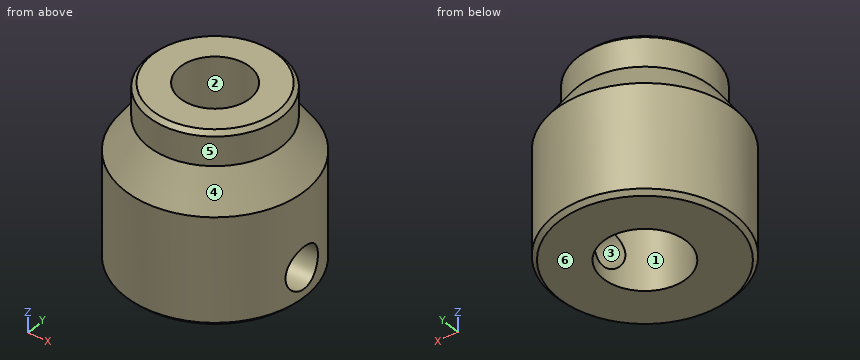
```python
from build123d import *

# Parameters (mm, degrees)
CONNECTOR_M5X0_8_TAPPED_HOLE_D        = 4.2
CONNECTOR_M5X0_8_TAPPED_HOLE_DEPTH    = 7.4
CONNECTOR_M5X0_8_TAPPED_HOLE_TIP      = 1.2618073
SET_SCREW_1_M3X0_5_TAPPED_HOLE_REACH  = 16.767
SET_SCREW_1_M3X0_5_TAPPED_HOLE_BORE_R = 1.25
EDGE_CHAMFERS_SIZE                    = 0.25


with BuildPart() as part:
    # Body Sketch → Body Revolve (revolve)
    with BuildSketch(Plane(origin=(0, 0, 0), x_dir=(-1, 0, 0), z_dir=(0, 1, 0))):
        Polygon((1, 10.5), (4, 10.5), (4, 8.5), (5.4, 6.5), (5.4, 0), (2.5, 0), (2.5, 6), (1, 6), align=None)
    revolve(axis=Axis((0, 0, 0), (0, 0, 1)))

    # Connector M5x0.8 Tapped Hole
    with Locations(Plane.XY.offset(10.5)):
        with Locations((0, 0)):
            Hole(CONNECTOR_M5X0_8_TAPPED_HOLE_D / 2, depth=CONNECTOR_M5X0_8_TAPPED_HOLE_DEPTH)
            with Locations((0, 0, -(CONNECTOR_M5X0_8_TAPPED_HOLE_DEPTH + CONNECTOR_M5X0_8_TAPPED_HOLE_TIP / 2))):  # 118° drill point
                Cone(0, CONNECTOR_M5X0_8_TAPPED_HOLE_D / 2, CONNECTOR_M5X0_8_TAPPED_HOLE_TIP, mode=Mode.SUBTRACT)

    # Set Screw 1 M3x0.5 Tapped Hole bore (on position points) → Set Screw 1 M3x0.5 Tapped Hole (cut, up to next)
    with BuildSketch(Plane(origin=(5.4, 0, 2), x_dir=(0, 1, 0), z_dir=(1, 0, 0)), mode=Mode.PRIVATE) as set_screw_1_m3x0_5_tapped_hole_sk1:
        Circle(SET_SCREW_1_M3X0_5_TAPPED_HOLE_BORE_R)
    set_screw_1_m3x0_5_tapped_hole_tool1 = extrude(set_screw_1_m3x0_5_tapped_hole_sk1.sketch, amount=-SET_SCREW_1_M3X0_5_TAPPED_HOLE_REACH, mode=Mode.PRIVATE) & part.part
    add(set_screw_1_m3x0_5_tapped_hole_tool1.solids().sort_by_distance((5.4, 0, 2))[0], mode=Mode.SUBTRACT)

    # Edge Chamfers
    edge_chamfers_edges = [part.edges().sort_by_distance(p)[0] for p in [
        (5.4, 0, 0),
        (4, 0, 10.5),
    ]]
    chamfer(edge_chamfers_edges, length=EDGE_CHAMFERS_SIZE)


solid = part.part
```
Build history of the part. All positions in model axes, mm. Face numbers are marked on the shaded views. A direction names the side the tool comes from. Give positions to 0.01 mm unless a question says otherwise; leave off trailing zeros. Loops run counter-clockwise (first coordinate to the right, second up) from the corner with the lowest first, then second, coordinate; pieces in that order, holes last.
1) Band-saw the part on D-D on z = 2. List the corners of the cut face in (x, y).
Values follow:
outline: (2.17, -1.25) arc R2.5 cw (long way) to (2.17, 1.25) - (5.25, 1.25) arc R5.4 ccw (long way) to (5.25, -1.25) - close
2) Drop flat-ended pins along their axis: P1, Ø5, axis at x = -2.5, z = 2, coming from the +Y side; P2, Ø3, axis at y = -4, z = 1.5, coming from the +X side; P3, Ø1, axis at x = 3.5, y = -3.5, coming from the +Z side; P4, Ø6, axis at x = -4, z = 9.5, coming from the +Y side. Give the stop position or say it passes through.
Values follow:
P1: stops at y = 5.4
P2: stops at x = 4.79
P3: stops at z = 7.86
P4: stops at y = 4.47
3) Two-plate mould, pull along X, no slides. Class the marked faces 1, 2, 3 and 4: released by +X, released by -X, zero draft, split by the parting line, or undercut.
Values follow:
face 1: undercut
face 2: undercut
face 3: zero draft
face 4: split by the parting line
4) Band-saw the part on A-A on x = 0. List the corners of the cut face in (y, z), then the cut area to 3 significant figures.
Values follow:
outline: (-5.4, 0.25) - (-5.15, 0) - (-2.5, 0) - (-2.5, 6) - (-2.1, 6) - (-2.1, 10.5) - (-3.75, 10.5) - (-4, 10.25) - (-4, 8.5) - (-5.4, 6.5) - close; (2.1, 6) - (2.5, 6) - (2.5, 0) - (5.15, 0) - (5.4, 0.25) - (5.4, 6.5) - (4, 8.5) - (4, 10.25) - (3.75, 10.5) - (2.1, 10.5) - close
area: 56.0 mm2
5) 3-axis set-ups, long thin cutter, end or side, ignore diameter. For the marked faces 5 and 6: which of +Z, -Z, +X, -X, +Y, -Y reach the whole face in a straight line?
Values follow:
face 5: +Z
face 6: -Z, +X, -X, +Y, -Y
6) Probe line 1 along Y through (x, z) = (0, 9.45); line 2 along Z through (x, y) = (3, 0); line 3 along Y through (x, z) = (4.45, 2). List the from-to ranges inside material, lowest first.
Values follow:
line 1: y = -4 to -2.1, 2.1 to 4
line 2: z = 0 to 0.75, 3.25 to 10.5
line 3: y = -3.06 to -1.25, 1.25 to 3.06
7) Band-saw the part on B-B on z = 9.5. List the corners of the cut face in (x, y).
Values follow:
outline: circle Ø8 at (0, 0); hole circle Ø4.2 at (0, 0)
8) Band-saw the part on C-C on z = 6.25. List the corners of the cut face in (x, y), then the cut area to 3 significant figures.
Values follow:
outline: circle Ø10.8 at (0, 0); hole circle Ø4.2 at (0, 0)
area: 77.8 mm2
